from build123d import *
from build123d.topology import SkipClean

# Parameters (mm, degrees)
BOSS_EXTRUDE1_DEPTH = 4
BOSS_EXTRUDE2_DEPTH = 2.5
SKETCH3_R           = 7.95
CUT_EXTRUDE1_DEPTH  = 9.25
SKETCH4_R           = 2
CUT_EXTRUDE2_DEPTH  = 9.25
CUT_EXTRUDE3_DEPTH  = 3.25
FILLET1_R           = 2.36
CHAMFER1_SIZE       = 3.5
CHAMFER1_SIZE2      = 2.020725942
BOSS_EXTRUDE4_DEPTH = 4
FILLET4_R           = 2
BOSS_EXTRUDE5_START = 2.25
SKETCH11_R          = 11.95
BOSS_EXTRUDE5_DEPTH = 2.25
CUT_EXTRUDE4_START  = -2.25
SKETCH12_R          = 7.95
CUT_EXTRUDE4_DEPTH  = 2.25
FILLET5_R           = 2.38


with BuildPart() as part:
    # Sketch1 → Boss-Extrude1 (new body)
    with BuildSketch(Plane(origin=(0, 0, 0), x_dir=(1, 0, 0), z_dir=(0, 1, 0))):
        with BuildLine():
            Line((-13.29118379, 20.889836125), (-0.68999579, 20.889836125))
            Line((-0.68999579, 20.889836125), (-0.68999579, 26.09210312))
            Line((-0.68999579, 26.09210312), (12.01000421, 26.09210312))
            Line((12.01000421, 26.09210312), (12.01000421, -28.90789688))
            Line((12.01000421, -28.90789688), (-0.68999579, -28.90789688))
            Line((-0.68999579, -28.90789688), (-0.68999579, -23.705629885))
            Line((-0.68999579, -23.705629885), (-13.29118379, -23.705629885))
            ThreePointArc((-13.29118379, -23.705629885), (-35.588916795, -1.40789688), (-13.29118379, 20.889836125))
        make_face()
    extrude(amount=BOSS_EXTRUDE1_DEPTH)

    # Sketch2 → Boss-Extrude2 (add)
    with BuildSketch(Plane(origin=(0, 4, 0), x_dir=(1, 0, 0), z_dir=(0, 1, 0))):
        with BuildLine():
            Line((-13.29118379, 20.889836125), (-0.68999579, 20.889836125))
            Line((-0.68999579, 20.889836125), (-0.68999579, 16.987726462))
            ThreePointArc((-0.68999579, 16.987726462), (9.006549215, -1.40789688), (-0.68999579, -19.803520222))
            Line((-0.68999579, -19.803520222), (-0.68999579, -23.705629885))
            Line((-0.68999579, -23.705629885), (-13.29118379, -23.705629885))
            ThreePointArc((-13.29118379, -23.705629885), (-35.588916795, -1.40789688), (-13.29118379, 20.889836125))
        make_face()
    extrude(amount=BOSS_EXTRUDE2_DEPTH)

    # Sketch3 → Cut-Extrude1 (cut)
    with BuildSketch(Plane.XZ):
        with Locations(Location((-13.29118379, 1.40789688, 0), (0, 0, 270))):
            Circle(SKETCH3_R)
    extrude(amount=-CUT_EXTRUDE1_DEPTH, mode=Mode.SUBTRACT)

    # Sketch4 → Cut-Extrude2 (cut)
    with BuildSketch(Plane.XZ):
        with Locations(Location((3.31000421, 24.40789688, 0), (0, 0, 270))):
            Circle(SKETCH4_R)
        with Locations(Location((3.310004206, -21.59210312, 0), (0, 0, 270))):
            Circle(SKETCH4_R)
    extrude(amount=-CUT_EXTRUDE2_DEPTH, mode=Mode.SUBTRACT)

    # Sketch5 → Cut-Extrude3 (cut)
    with BuildSketch(Plane.XZ):
        with BuildLine():
            ThreePointArc((-20.917233099, -7.792422241), (-25.24118379, 1.40789688), (-20.917233099, 10.608216001))
            Line((-20.917233099, 10.608216001), (-24.193916765, 16.291878661))
            ThreePointArc((-24.193916765, 16.291878661), (-31.74118379, 1.40789688), (-24.193916765, -13.476084902))
            Line((-24.193916765, -13.476084902), (-20.917233099, -7.792422241))
        make_face()
        with BuildLine():
            Line((-20.729723635, 18.291931497), (-17.445869217, 12.612408873))
            ThreePointArc((-17.445869217, 12.612408873), (-7.31618379, 11.756900455), (-1.510449053, 3.412089752))
            Line((-1.510449053, 3.412089752), (5.05008903, 3.407949716))
            ThreePointArc((5.05008903, 3.407949716), (-4.06618379, 17.38606558), (-20.729723635, 18.291931497))
        make_face()
        with BuildLine():
            ThreePointArc((-1.510449053, -0.596295992), (-7.31618379, -8.941106696), (-17.445869217, -9.796615113))
            Line((-17.445869217, -9.796615113), (-20.729723635, -15.476137738))
            ThreePointArc((-20.729723635, -15.476137738), (-4.06618379, -14.57027182), (5.05008903, -0.592155956))
            Line((5.05008903, -0.592155956), (-1.510449053, -0.596295992))
        make_face()
    extrude(amount=-CUT_EXTRUDE3_DEPTH, mode=Mode.SUBTRACT)

    # Fillet1
    fillet1_edges = [part.edges().sort_by_distance(p)[0] for p in [
        (-20.917233099, 1.625, 10.608216001),
        (-20.917233099, 1.625, -7.792422241),
        (-24.193916765, 1.625, -13.476084902),
        (-24.193916765, 1.625, 16.291878661),
        (5.05008903, 1.625, 3.407949716),
        (-1.510449053, 1.625, 3.412089752),
        (-20.729723635, 1.625, 18.291931497),
        (-1.510449053, 1.625, -0.596295992),
        (5.05008903, 1.625, -0.592155956),
        (-20.729723635, 1.625, -15.476137738),
    ]]
    fillet(fillet1_edges, radius=FILLET1_R)

    # Chamfer1
    chamfer1_edges = [part.edges().sort_by_distance(p)[0] for p in [
        (12.01000421, 0, 1.40789688),
    ]]
    chamfer1_side = [part.faces().sort_by_distance(p)[0] for p in [
        (-3.702499267, 0, 18.015985651),
    ]]
    chamfer(chamfer1_edges, length=CHAMFER1_SIZE, length2=CHAMFER1_SIZE2, reference=chamfer1_side[0])

    # Sketch10 → Boss-Extrude4 (add)
    with BuildSketch(Plane.XZ):
        with BuildLine():
            Line((-0.68999579, -22.889836125), (-13.29118379, -22.889836125))
            ThreePointArc((-13.29118379, -22.889836125), (-37.588916795, 1.40789688), (-13.29118379, 25.705629885))
            Line((-13.29118379, 25.705629885), (-0.68999579, 25.705629885))
            Line((-0.68999579, 25.705629885), (-0.68999579, 23.705629885))
            Line((-0.68999579, 23.705629885), (-13.29118379, 23.705629885))
            ThreePointArc((-13.29118379, 23.705629885), (-35.588916795, 1.40789688), (-13.29118379, -20.889836125))
            Line((-13.29118379, -20.889836125), (-0.68999579, -20.889836125))
            Line((-0.68999579, -20.889836125), (-0.68999579, -22.889836125))
        make_face()
    extrude(amount=-BOSS_EXTRUDE4_DEPTH)

    # Fillet4
    fillet4_edges = [part.edges().sort_by_distance(p)[0] for p in [
        (-6.99058979, 0, 25.705629885),
        (-37.588916795, 0, 1.40789688),
        (-6.99058979, 0, -22.889836125),
    ]]
    fillet(fillet4_edges, radius=FILLET4_R)

    # Sketch11 → Boss-Extrude5 (add)
    with SkipClean():  # the faces are left unmerged after this step: merging them gives an invalid solid
        with BuildSketch(Plane.XZ.offset(BOSS_EXTRUDE5_START)):
            with Locations(Location((-13.29118379, 1.40789688, 0), (0, 0, 270))):
                Circle(SKETCH11_R)
        extrude(amount=-BOSS_EXTRUDE5_DEPTH)

    # Sketch12 → Cut-Extrude4 (cut)
    with SkipClean():  # the faces are left unmerged after this step: merging them gives an invalid solid
        with BuildSketch(Plane(origin=(0, 0, 0), x_dir=(1, 0, 0), z_dir=(0, 1, 0)).offset(CUT_EXTRUDE4_START)):
            with Locations(Location((-13.29118379, -1.40789688, 0), (0, 0, 270))):
                Circle(SKETCH12_R)
        extrude(amount=CUT_EXTRUDE4_DEPTH, mode=Mode.SUBTRACT)

    # Fillet5
    fillet5_edges = [part.edges().sort_by_distance(p)[0] for p in [
        (-0.68999579, 5.25, 19.803520222),
        (-0.68999579, 5.25, -16.987726462),
    ]]
    fillet(fillet5_edges, radius=FILLET5_R)


solid = part.part
Geometry check sheet. Reference: the model listing, model coordinates, mm. A direction names the side the tool comes from. Coordinates: 2 decimals unless noted, no trailing zeros. Loops run counter-clockwise (first coordinate to the right, second up) from the corner with the lowest first, then second, coordinate; pieces in that order, holes last. Notation, with made-up numbers: (83.5, -38.5) - (128.5, -38.5) arc R16 cw to (128.5, -7.5) - close; hole circle Ø1 at (-22, -3). An arc over 180 degrees is marked (long way). Use one line per item in the form item = value. Start each with the question number.
Item 1: Thickness scan on probe 1 along Z at (x, y) = (-14, 2.75); probe 2 along Z at (x, y) = (5, 0.25); probe 3 along Y at (x, z) = (-30.5, 14). Record the ranges inside material, lowest first.
Item 2: Section check C-C, the plane y = -0.75. Enter the section's corners in (x, z).
Item 3: Mould release check, pull along X, two halves, no side actions. Record for faces 1 (the face through (-21.54, 1.65, -7.94)), 2 (the face through (-27, 3.25, 2)), 3 (the face through (9.005, 5.232, 1.121)), 4 (the face through (6, 2, 28.908)): +X half, -X half, draft (parallel to the pull), parting line (faces both ways), or undercut.
Item 4: Tool access check on faces 5 (the face through (-8, 3.25, 14)), 6 (the face through (-23, 6.5, 1)), 7 (the face through (-0.437, 5.268, 19.949)), 8 (the face through (-6.902, 0.57, 25.104)), 9 (the face through (-0.45, 5.27, -17.16)). Record the directions out of +Z, -Z, +X, -X, +Y, -Y that give a thin tool (end or side, any length) a straight path to the whole face; none if there is none.
Item 5: Section check A-A, the plane y = 5.75. Enter the section's corners in (x, z).
Item 6: Section check B-B, the plane x = 7.5. Enter the section's corners in (y, z), and give its area (3 significant figures).
Item 7: Gauge pin test, flat ends, axial feed: pin 1 (0.8 mm diameter, centred on x = -5, y = 5, fed in from -Z); pin 2 (12 mm diameter, centred on x = -20, z = -20, fed in from -Y); pin 3 (2 mm diameter, centred on x = -2, y = 0.5, fed in from +Z). Record the tip position at first contact, or that the pin passes through.
Computed:
q1.probe_1 = -22.88 to -17.03, -10.52 to -6.51, 9.33 to 13.34, 19.84 to 25.7
q1.probe_2 = -26.09 to -22.66, -20.52 to 23.34, 25.48 to 28.91
q1.probe_3 = 0 to 6.5
q2.outline = circle Ø23.9 at (-13.29, 1.41); hole circle Ø15.9 at (-13.29, 1.41)
q3.face_1 = undercut
q3.face_2 = undercut
q3.face_3 = +X half
q3.face_4 = draft
q4.face_5 = -Y
q4.face_6 = +Z, -Z, +X, -X, +Y
q4.face_7 = +Z, +X, +Y
q4.face_8 = +Z, -X, -Y
q4.face_9 = -Z, +X, +Y
q5.outline = (-13.29, -20.89) - (-0.69, -20.89) - (-0.69, -18.2) arc R2.38 cw to (0.25, -16.31) arc R22.3 ccw to (0.25, 19.13) arc R2.38 cw to (-0.69, 21.02) - (-0.69, 23.71) - (-13.29, 23.71) arc R22.3 ccw to start; hole circle Ø15.9 at (-13.29, 1.41)
q6.outline = (0, -26.09) - (4, -26.09) - (4, -6.65) - (6.5, -6.65) - (6.5, 9.46) - (4, 9.46) - (4, 28.91) - (0, 28.91) - close
q6.area = 260 mm2
q7.pin_1 = -20.89
q7.pin_2 = 0
q7.pin_3 = 25.64
